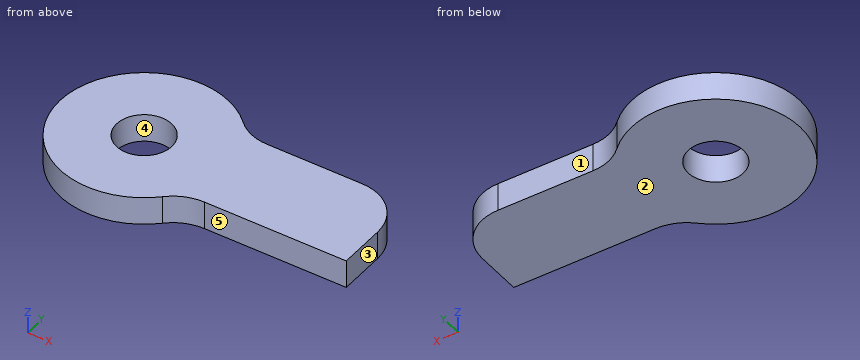
Autodesk Inventor part; units mm, degrees
ref_plane "YZ Plane" through (0, 0, 0) normal (1, 0, 0) x (0, 1, 0)
ref_plane "XZ Plane" through (0, 0, 0) normal (0, 1, 0) x (-1, 0, 0)
ref_plane "XY Plane" through (0, 0, 0) normal (0, 0, 1) x (1, 0, 0)
sketch "Sketch1" plane through (0, 0, 0) normal (0, 0, 1) x (1, 0, 0)
  line L0 (0, 0) -> (30, 0)
  line L1 (30, 0) -> (30, 10)
  line L2 (30, 10) -> (0, 10)
  line L3 (0, 10) -> (0, 0)
  dimension "d0" = 30
  dimension "d1" = 10
extrude "Extrusion1" add sketch "Sketch1" along normal blind 3
sketch "Sketch2" plane through (0, 0, 3) normal (0, 0, 1) x (1, 0, 0)
  line L0 (30, 10) -> (0, 10)
  line L1 (0, 0) -> (30, 0)
  line L2 (0, 10) -> (0, 0)
  point P0 (5, 5)
  dimension "d4" = 5
  dimension "d5" = 5
  dimension "d6" = 5
hole "Hole1" at (5, 5, 3) direction (0, 0, -1) diameter 5.9 end through all
fillet "Fillet2" radius 5 1 edges at (30, 10, 1.5)
sketch "Sketch4" plane through (0, 0, 3) normal (0, 0, 1) x (1, 0, 0)
  circle A0 centre (5, 5) radius 2.95
  circle A1 centre (5, 5) radius 9
  circle A2 centre (5, 5) radius 2.95
  point P0 (0, 0)
  dimension "d16" = 18
extrude "Extrusion2" add sketch "Sketch4" against normal up to surface (3 mm away)
fillet "Fillet3" radius 5 2 edges at (12.4833, 10, 1.5) (12.4833, 0, 1.5)
properties part number "Selection_Lever 2" material "Nylon 6/6"
CAD build for the part. Positions are in the model's coordinates, mm. Face numbers are marked on the shaded views. A direction names the side the tool comes from. Round coordinates to 2 decimals unless told otherwise and drop trailing zeros. Loops run counter-clockwise (first coordinate to the right, second up) from the corner with the lowest first, then second, coordinate; pieces in that order, holes last.
(1) Wall check: line 1 along X through (y, z) = (5, 2); line 2 along Y through (x, z) = (21.5, 2.3); line 3 along X through (y, z) = (11, 2.4). Give the ranges that are in metal, low to high.
(2) Two-plate mould, pull along X, no slides. Class the marked faces 3, 4 and 5: +X half, -X half, draft (parallel to the pull), parting line (faces both ways), or undercut.
(3) Which spindle directions (+Z, -Z, +X, -X, +Y, -Y) get a long thin tool onto all of the face, cutting with end or side? Do the marked faces 1 and 2. Say none if no direction does.
(4) Cut at B-B (z = 1.4). Give the cut face in (x, y), plus the area to 3 significant figures.
(5) Cut at D-D (x = 28). Give the cut face in (y, z), plus the area to 3 significant figures.
(6) Cut at C-C (y = 7.5). Give the cut face in (x, z).
(7) Drop flat-ended pins along their axis: pin 1 (7 mm diameter, centred on x = 5, y = 5, fed in from -Z); pin 2 (1 mm diameter, centred on x = 8.5, z = 2, fed in from +Y); pin 3 (1 mm diameter, centred on x = 13, z = 1.5, fed in from -Y). Give the stop position or say it passes through.
(8) Cut at A-A (x = 5). Give the cut face in (y, z), plus the area to 3 significant figures.
Findings below:
1. line 1: x = -4 to 2.05, 7.95 to 30
1. line 2: y = 0 to 10
1. line 3: x = -1.71 to 11.8
2. face 3: +X half
2. face 4: undercut
2. face 5: draft
3. face 1: +Z, -Z, +X, +Y
3. face 2: -Z, +X, -X, +Y, -Y
4. outline: (11.3, -1.43) arc R5 cw to (14.8, 0) - (30, 0) - (30, 5) arc R5 ccw to (25, 10) - (14.8, 10) arc R5 cw to (11.3, 11.43) arc R9 ccw (long way) to start; hole circle Ø5.9 at (5, 5)
4. area: 388 mm2
5. outline: (0, 0) - (9, 0) - (9, 3) - (0, 3) - close
5. area: 27.0 mm2
6. outline: (-3.65, 0) - (3.43, 0) - (3.43, 3) - (-3.65, 3) - close; (6.57, 0) - (29.33, 0) - (29.33, 3) - (6.57, 3) - close
7. pin 1: stops at z = 0
7. pin 2: stops at y = 13.49
7. pin 3: stops at y = -0.56
8. outline: (-4, 0) - (2.05, 0) - (2.05, 3) - (-4, 3) - close; (7.95, 0) - (14, 0) - (14, 3) - (7.95, 3) - close
8. area: 36.3 mm2
